Check sheet for the modelled part. Datum: model origin and axes. Units: mm. Face numbers are marked on the shaded views. A direction names the side the tool comes from. Round coordinates to 2 decimals unless told otherwise and drop trailing zeros. Write each loop counter-clockwise with the first axis right and the second up, starting at its lowest first coordinate (ties: lowest second). Pieces come first, ordered by that corner, then holes. Notation, with made-up numbers: (89.5, 16) -> (140.5, 16) arc R21 ccw to (140.5, 52) -> close; hole circle Ø10 at (-5, 35). An arc over 180 degrees is marked (long way). One line per item, written item: value.
from build123d import *

# Parameters (mm, degrees)
F1_DEPTH = 10


with BuildPart() as f1:
    # F0 (on Front) → F1 (new body)
    with BuildSketch(Plane.XZ):
        with BuildLine():
            ThreePointArc((60, 13), (59.414214, 14.414214), (58, 15))
            Line((58, 15), (-58, 15))
            ThreePointArc((-58, 15), (-59.414214, 14.414214), (-60, 13))
            Line((-60, 13), (-60, -13))
            ThreePointArc((-60, -13), (-59.414214, -14.414214), (-58, -15))
            Line((-58, -15), (58, -15))
            ThreePointArc((58, -15), (59.414214, -14.414214), (60, -13))
            Line((60, -13), (60, 13))
        make_face()
        with BuildLine():
            Line((-44.987983, 5), (45.101259, 5))
            ThreePointArc((45.101259, 5), (48.636793, 3.535534), (50.101259, 0))
            ThreePointArc((50.101259, 0), (48.636793, -3.535534), (45.101259, -5))
            Line((45.101259, -5), (-44.987983, -5))
            ThreePointArc((-44.987983, -5), (-49.987983, 0), (-44.987983, 5))
        make_face(mode=Mode.SUBTRACT)
    extrude(amount=F1_DEPTH)


solid = f1.part
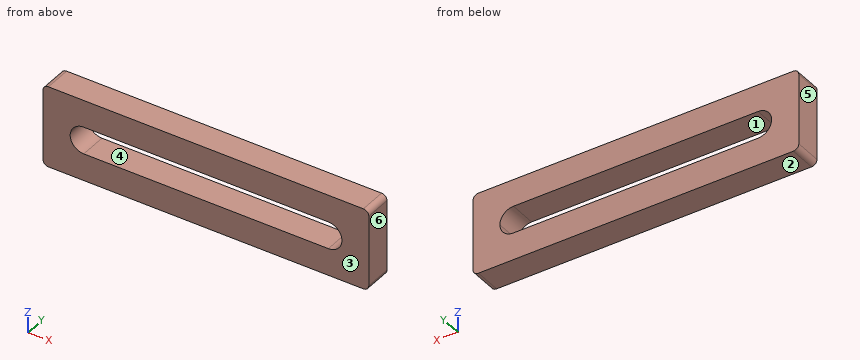
Item 1: Mould release check, pull along X, two halves, no side actions. Record for the marked faces 3, 4, 5 and 6: pulls with the +X half, pulls with the -X half, needs draft (parallel to the pull), parting line crosses it, or undercut.
Answer:
face 3: needs draft
face 4: undercut
face 5: pulls with the -X half
face 6: pulls with the +X half
Item 2: Sectioned sample at B-B on x = -29. Enter the section's corners in (y, z), and give its area (3 significant figures).
Answer:
outline: (-10, -15) -> (0, -15) -> (0, -5) -> (-10, -5) -> close; (-10, 5) -> (0, 5) -> (0, 15) -> (-10, 15) -> close
area: 200 mm^2
Item 3: Thickness scan on line 1 (Z direction, x = -16.5, y = -2.5); line 2 (X direction, y = -4.75, z = 0.5); line 3 (Z direction, x = 46, y = -6). Record the ranges inside material, lowest first.
Answer:
line 1: z = -15 to -5, 5 to 15
line 2: x = -60 to -49.96, 50.08 to 60
line 3: z = -15 to -4.92, 4.92 to 15
Item 4: Sectioned sample at A-A on y = -3.75. Enter the section's corners in (x, z).
Answer:
outline: (-60, -13) arc R2 ccw to (-58, -15) -> (58, -15) arc R2 ccw to (60, -13) -> (60, 13) arc R2 ccw to (58, 15) -> (-58, 15) arc R2 ccw to (-60, 13) -> close; hole (-44.99, -5) -> (45.1, -5) arc R5 ccw to (45.1, 5) -> (-44.99, 5) arc R5 ccw to start
Item 5: Sectioned sample at C-C on z = -2.5. Enter the section's corners in (x, y), and give its area (3 significant figures).
Answer:
outline: (-60, -10) -> (-49.32, -10) -> (-49.32, 0) -> (-60, 0) -> close; (49.43, -10) -> (60, -10) -> (60, 0) -> (49.43, 0) -> close
area: 213 mm^2
Item 6: Tool access check on the marked faces 1 and 2. Record the directions out of +Z, -Z, +X, -X, +Y, -Y that give a thin tool (end or side, any length) a straight path to the whole face; none if there is none.
Answer:
face 1: +Y, -Y
face 2: -Z, +X, -X, +Y, -Y
